Part model, mm, in its own coordinate system. Face numbers are marked on the shaded views. A direction names the side the tool comes from. Round coordinates to 2 decimals unless told otherwise and drop trailing zeros. Loops run counter-clockwise (first coordinate to the right, second up) from the corner with the lowest first, then second, coordinate; pieces in that order, holes last. Notation, with made-up numbers: (-11.5, -11) -> (39.5, -11) arc R17 cw to (39.5, -1) -> close; hole circle Ø11 at (27.5, -37). An arc over 180 degrees is marked (long way). Use a Markdown table: item, result. Add a question column.
Item 1: Probe line 1 (Z direction, x = 2.25, y = -0.25); line 2 (Z direction, x = 11, y = -0.5); line 3 (X direction, y = -0.15, z = -0.3). List the from-to ranges inside material, lowest first. Write a range as [from, to].
Item 2: Cut at B-B, the plane x = 7.5. List the corners of the cut face in (y, z).
Item 3: Which spindle directions (+Z, -Z, +X, -X, +Y, -Y) get a long thin tool onto all of the face, cutting with end or side? Do the marked faces 1 and 2. Say none if no direction does.
Item 4: Cut at C-C, the plane x = -1.5. List the corners of the cut face in (y, z).
Item 5: Two-plate mould, pull along Z, no slides. Class the marked faces 3 and 4: pulls with the +Z half, pulls with the -Z half, needs draft (parallel to the pull), parting line crosses it, or undercut.
Item 6: Cut at A-A, the plane z = -0.1. List the corners of the cut face in (x, y).
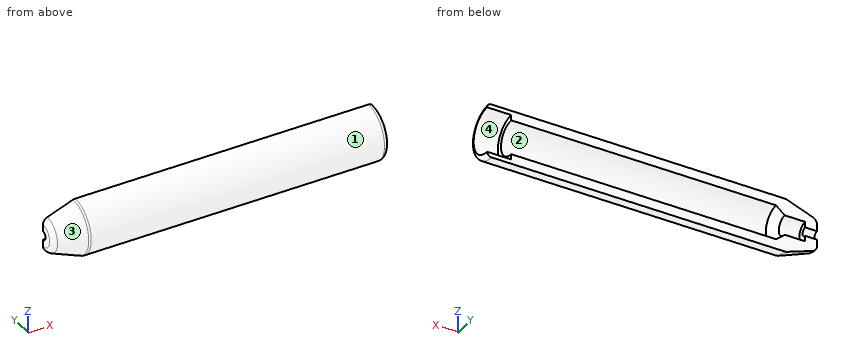
```python
from build123d import *

# Parameters (mm, degrees)
REVOLVE1_ANGLE = 180


with BuildPart() as part:
    # Sketch1 → Revolve1 (revolve)
    with BuildSketch(Plane(origin=(0, 0, 0), x_dir=(1, 0, 0), z_dir=(0, 1, 0))):
        with BuildLine():
            Line((-2.426089026, 0.9), (-1.253621619, 1.331536072))
            ThreePointArc((-1.253621619, 1.331536072), (-1.202626886, 1.345347949), (-1.15, 1.35))
            Line((-1.15, 1.35), (12.217609628, 1.35))
            ThreePointArc((12.217609628, 1.35), (12.359030984, 1.291421356), (12.417609628, 1.15))
            Line((12.417609628, 1.15), (11.317609628, 1.15))
            Line((11.317609628, 1.15), (11.317609628, 0.9))
            Line((11.317609628, 0.9), (3.617609628, 0.9))
            Line((3.617609628, 0.9), (2.917609628, 0.9))
            Line((2.917609628, 0.9), (-0.754449261, 0.9))
            Line((-0.754449261, 0.9), (-1.15, 0.56))
            Line((-1.15, 0.56), (-2.082390372, 0.56))
            Line((-2.082390372, 0.56), (-2.082390372, 0.3))
            Line((-2.082390372, 0.3), (-2.622467407, 0.3))
            Line((-2.622467407, 0.3), (-2.622467407, 0.618463928))
            ThreePointArc((-2.622467407, 0.618463928), (-2.568522772, 0.790093637), (-2.426089026, 0.9))
        make_face()
    revolve(axis=Axis((-3.185032955, 0, -0.1), (-1, 0, 0)), revolution_arc=REVOLVE1_ANGLE)


solid = part.part
```
A:
| question | item | result |
|---|---|---|
| 1 | line 1 | z = [-1.32, -0.86], [0.66, 1.12] |
| 1 | line 2 | z = [-1.25, -0.72], [0.52, 1.05] |
| 1 | line 3 | x = [-2.62, -2.08] |
| 2 | outline | (0, -1.35) -> (0, -0.9) arc R0.8 cw to (0, 0.7) -> (0, 1.15) arc R1.25 ccw to start |
| 3 | face 1 | +X, -X, -Y |
| 3 | face 2 | +X, +Y |
| 4 | outline | (0, -1.24) -> (0, -0.56) arc R0.46 cw to (0, 0.36) -> (0, 1.04) arc R1.14 ccw to start |
| 5 | face 3 | parting line crosses it |
| 5 | face 4 | undercut |
| 6 | outline | (-2.62, -0.52) arc R0.3 ccw to (-2.43, -0.8) -> (-1.25, -1.23) arc R0.3 ccw to (-1.15, -1.25) -> (12.22, -1.25) arc R0.2 ccw to (12.42, -1.05) -> (11.32, -1.05) -> (11.32, -0.8) -> (-0.75, -0.8) -> (-1.15, -0.46) -> (-2.08, -0.46) -> (-2.08, -0.2) -> (-2.62, -0.2) -> close |
